```python
from build123d import *

# Parameters (mm, degrees)
F0_R     = 5.5
F1_DEPTH = 9
F3_DEPTH = 9
F4_R     = 7
F5_DEPTH = 9


with BuildPart() as f1:
    # F0 (on Top) → F1 (new body)
    with BuildSketch(Plane.XY):
        with BuildLine():
            Line((46, 24), (-13, 24))
            Line((-13, 24), (-13, 0))
            ThreePointArc((-13, 0), (-9.192388, -9.192388), (0, -13))
            Line((0, -13), (33, -13))
            ThreePointArc((33, -13), (42.192388, -9.192388), (46, 0))
            Line((46, 0), (46, 24))
        make_face()
        Circle(F0_R, mode=Mode.SUBTRACT)
        with Locations((33, 0)):
            Circle(F0_R, mode=Mode.SUBTRACT)
    extrude(amount=F1_DEPTH)

    # F2 (on face) → F3 (join)
    with BuildSketch(Plane(origin=(0, 24, 0), x_dir=(-1, 0, 0), z_dir=(0, 1, 0))):
        Polygon((-46, 9), (13, 9), (-53.313708, 75.313708), (-75.941125, 52.686292), (-46, 0), align=None)
    extrude(amount=-F3_DEPTH)

    # F4 (on face) → F5 (join)
    with BuildSketch(Plane(origin=(64.313708, 0, 64.313708), x_dir=(0, 1, 0), z_dir=(0.707107, 0, 0.707107))):
        with BuildLine():
            Line((24, -16.443651), (24, 15.556349))
            Line((24, 15.556349), (-5, 15.556349))
            ThreePointArc((-5, 15.556349), (-21, -0.443651), (-5, -16.443651))
            Line((-5, -16.443651), (24, -16.443651))
        make_face()
        with Locations((-5, -0.443651)):
            Circle(F4_R, mode=Mode.SUBTRACT)
    extrude(amount=F5_DEPTH)


solid = f1.part
```
Geometry: final body of the model. Coordinates: model frame, mm. A direction names the side the tool comes from. Give positions to 0.01 mm unless a question says otherwise; leave off trailing zeros. Write each loop counter-clockwise with the first axis right and the second up, starting at its lowest first coordinate (ties: lowest second). Pieces come first, ordered by that corner, then holes.
1. Section query D-D, the plane y = -2.5. Return loops of the section in (x, z), then the cut area to 3 significant figures.
2. Line query: probe 1 along Y at (x, z) = (33, 2.25); probe 2 along Z at (x, y) = (32, -6.5); probe 3 along Y at (x, z) = (24.5, 43). Output: solid intervals per line, ascending.
3. Pin query (flat end, axial travel): P1, Ø10, axis at y = 7.5, z = 43, coming from the -X side; P2, Ø10, axis at x = 33.5, y = 8, coming from the +Z side; P3, Ø2.5, axis at y = 10, z = 4, coming from the +X side; P4, Ø8, axis at y = 9, z = 71, coming from the -X side. Return the tip coordinate at first contact, or that it passes through.
4. Section query C-C, the plane y = -10. Return loops of the section in (x, z), then the cut area to 3 significant figures.
5. Reachability of faces 4 (the flat face through (16, 1, 9)), 5 (the flat face through (46, 7, 4)), 6 (the cylindrical face through (27.505, 0.242, 4.437)) from +Z, -Z, +X, -X, +Y, -Y: full face, straight path, thin tool, end or side. Return the list, or none.
6. Section query B-B, the plane x = 29. Return loops of the section in (y, z).
7. Section query A-A, the plane y = 13.5. Return loops of the section in (x, z), then the cut area to 3 significant figures.
8. Draft query along Z for faces 1 (the cylindrical face through (62.86, -5.91, 72.05)), 2 (the flat face through (61.955, 1.185, 66.673)), 3 (the flat face through (-13, 12, 4)). Return one class per face: released by +Z, released by -Z, zero draft, split by the parting line, or undercut.
Computed:
1. outline: (-12.76, 0) - (-4.9, 0) - (-4.9, 9) - (-12.76, 9) - close; (4.9, 0) - (28.1, 0) - (28.1, 9) - (4.9, 9) - close; (37.9, 0) - (45.76, 0) - (45.76, 9) - (37.9, 9) - close; (53.31, 75.31) - (60, 68.62) - (66.37, 74.99) - (59.68, 81.68) - close; (69.25, 59.38) - (75.94, 52.69) - (82.31, 59.05) - (75.61, 65.74) - close
1. area: 521 mm2
2. probe 1: y = -13 to -5.5, 5.5 to 24
2. probe 2: z = 0 to 9
2. probe 3: y = 15 to 24
3. P1: passes through
3. P2: stops at z = 9
3. P3: stops at x = 46
3. P4: stops at x = 53.63
4. outline: (-8.31, 0) - (41.31, 0) - (41.31, 9) - (-8.31, 9) - close; (53.88, 74.75) - (61.16, 67.46) - (67.53, 73.83) - (60.24, 81.11) - close; (68.09, 60.54) - (75.37, 53.25) - (81.74, 59.62) - (74.46, 66.9) - close
4. area: 632 mm2
5. face 4: +Z, +X, -X, -Y
5. face 5: +Z, -Z, +X, -Y
5. face 6: +Z, -Z
6. outline: (-13, 0) - (-3.77, 0) - (-3.77, 9) - (-13, 9) - close; (3.77, 0) - (24, 0) - (24, 51) - (15, 51) - (15, 9) - (3.77, 9) - close
7. outline: (-13, 0) - (46, 0) - (46, 9) - (-13, 9) - close; (53.31, 75.31) - (75.94, 52.69) - (82.31, 59.05) - (59.68, 81.68) - close
7. area: 819 mm2
8. face 1: undercut
8. face 2: released by -Z
8. face 3: zero draft
